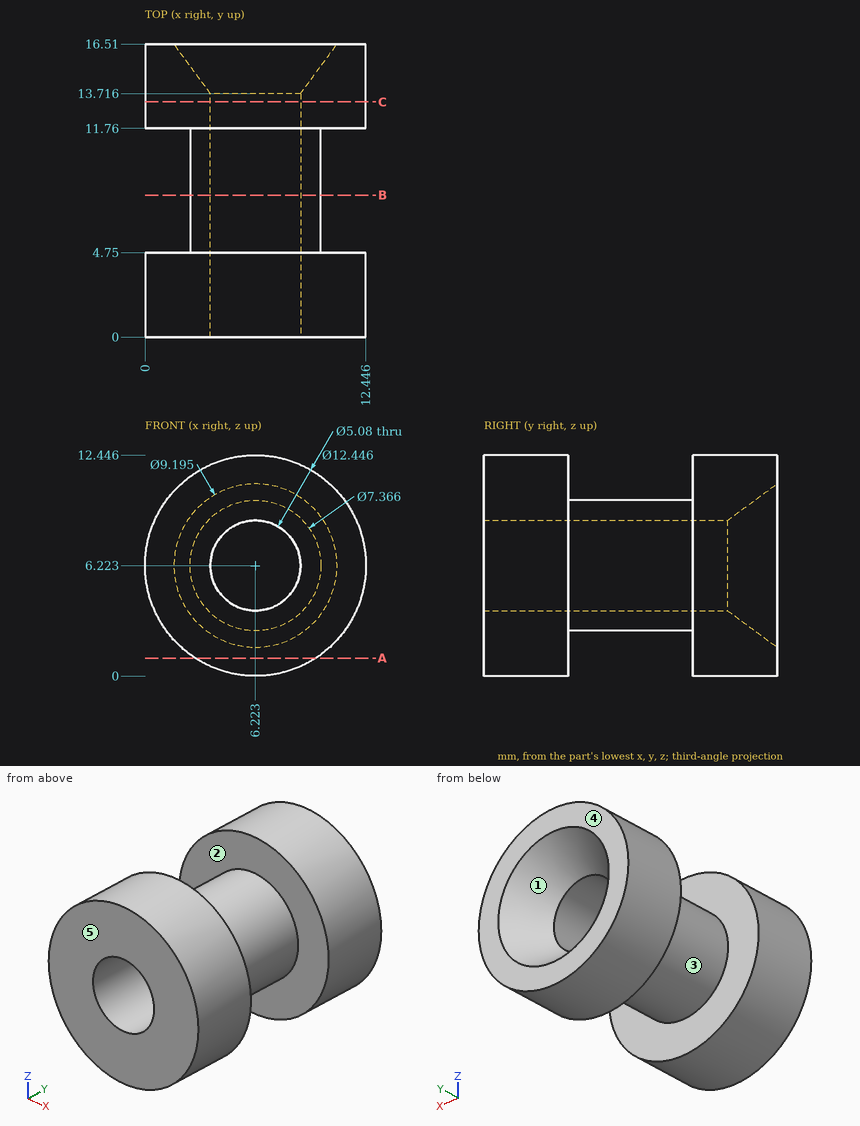
Input: dimensioned drawing with shaded views. Units: mm. Origin: part minimum x, y, z. A direction names the side the tool comes from. Round coordinates to 2 decimals unless told otherwise and drop trailing zeros. Order: outer loops, then holes, each group sorted by start corner. A loop starts at its lowest first (then second) coordinate and runs counter-clockwise, first axis right, second up. Notation, with made-up numbers: (39.5, 27) - (64.5, 27) arc R18 cw to (64.5, 47) - close; hole circle Ø5 at (-11.75, -27.5). An arc over 180 degrees is marked (long way). Answer as a JSON object with one key per item and string values. Group by question number.
(1) Cut plane A-A (z = 1). Return loops of the section in (x, y).
(2) Pin query (flat end, axial travel): P1, Ø1.5, axis at x = 7.5, y = 8.5, coming from the -Z side; P2, Ø1, axis at y = 14, z = 8.5, coming from the +X side; P3, Ø1, axis at x = 3.5, y = 2, coming from the +Z side (1 decimal). Return the tip coordinate at first contact, or that it passes through.
(3) Cut plane B-B (y = 8). Return loops of the section in (x, z).
(4) Cut plane C-C (y = 13.25). Return loops of the section in (x, z).
(5) Material intervals for probe 1 along Y at (x, z) = (1.5, 5); probe 2 along X at (y, z) = (9, 6.25); probe 3 along X at (y, z) = (1.5, 4.5), sorted ascending. Write a range as from..to.
(6) Reachability of the marked faces 1 and 2 from +Z, -Z, +X, -X, +Y, -Y: full face, straight path, thin tool, end or side. Return the list, or none.
(7) Draft query along Y for the marked faces 3, 4 and 5. Return one class per face: released by +Y, released by -Y, zero draft, split by the parting line, or undercut.
Here are the results:
{
 "1": {"outline": "(2.84, 0) - (9.61, 0) - (9.61, 4.75) - (2.84, 4.75) - close; (2.84, 11.76) - (9.61, 11.76) - (9.61, 16.51) - (2.84, 16.51) - close"},
 "2": {"P1": "stops at z = 2.58", "P2": "stops at x = 12.19", "P3": "stops at z = 12"},
 "3": {"outline": "circle Ø7.37 at (6.22, 6.22); hole circle Ø5.08 at (6.22, 6.22)"},
 "4": {"outline": "circle Ø12.45 at (6.22, 6.22); hole circle Ø5.08 at (6.22, 6.22)"},
 "5": {"probe 1": "y = 0..4.75, 11.76..16.51", "probe 2": "x = 2.54..3.68, 8.76..9.91", "probe 3": "x = 0.24..4.36, 8.09..12.2"},
 "6": {"face 1": "+Y", "face 2": "none"},
 "7": {"face 3": "undercut", "face 4": "released by +Y", "face 5": "released by -Y"}
}
